Source: CAD feature listing. Evaluate the final solid. Frame: model axes, mm. Face numbers are marked on the shaded views. A direction names the side the tool comes from. Give positions to 0.01 mm unless a question says otherwise; leave off trailing zeros. Loops run counter-clockwise (first coordinate to the right, second up) from the corner with the lowest first, then second, coordinate; pieces in that order, holes last. Notation, with made-up numbers: M 16.5,-29.5 L 39.5,-29.5 A19 cw 39.5,-17.5 Z; hole C 28,77 d6. An arc over 180 degrees is marked long. Write item = value, one per line.
Solid Edge part; units mm, degrees
sketch "Sketch1" plane through (0, 0, 0) normal (0, 0, 1) x (1, 0, 0)
  circle A0 centre (0, 0) radius 3
extrude "Protrusion1" add sketch "Sketch1" along normal blind 37
sketch "Sketch2" plane through (0, 0, 37) normal (0, 0, 1) x (1, 0, 0)
  line L0 (-2.8847, 4.9965) -> (-5.7695, 0)
  line L1 (-5.7695, 0) -> (-2.8847, -4.9965)
  line L2 (-2.8847, -4.9965) -> (2.8847, -4.9965)
  line L3 (2.8847, -4.9965) -> (5.7695, 0)
  line L4 (5.7695, 0) -> (2.8847, 4.9965)
  line L5 (2.8847, 4.9965) -> (-2.8847, 4.9965)
extrude "ExtrudedProtrusion_2" add sketch "Sketch2" along normal blind 4
cosmetic_thread "Thread_1" thread depth 10
properties material "Steel"
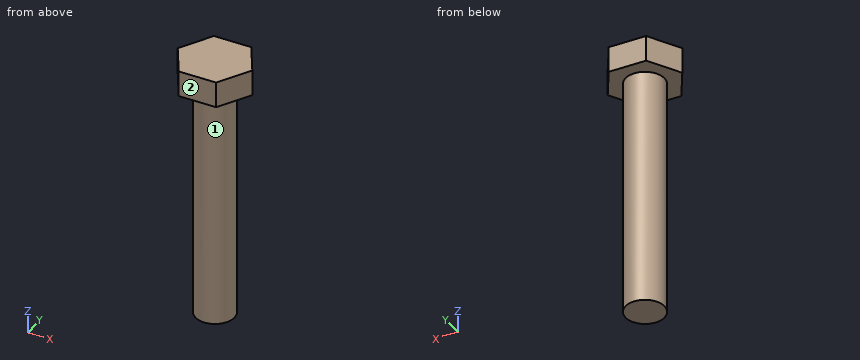
1. Cut plane D-D, the plane x = 5.25. Return the cut outline in (y, z), then the cut area to 3 significant figures.
Derived:
outline = M -0.9,37 L 0.9,37 L 0.9,41 L -0.9,41 Z
area = 7.20 mm²
2. Material intervals for probe 1 along Y at (x, z) = (0, 9); probe 2 along Z at (x, y) = (0.5, -3.25); probe 3 along X at (y, z) = (-2.75, 7.5), sorted ascending. Write a range as from..to.
Derived:
probe_1 = -3..3
probe_2 = 37..41
probe_3 = -1.2..1.2
3. First-contact query: pin 1 Ø4 at (x, z) = (-3.5, 14) entering from +Y; pin 2 Ø5 at (x, z) = (-3.5, 7) entering from -Y; pin 3 Ø1 at (y, z) = (0, 5.5) entering from -X. Flat tips, straight axial feed; report the tip coordinate or a pass-through.
Derived:
pin_1 = 2.6
pin_2 = -2.83
pin_3 = -3
4. Reachability of the marked faces 1 and 2 from +Z, -Z, +X, -X, +Y, -Y: full face, straight path, thin tool, end or side. Return the list, or none.
Derived:
face_1 = -Z
face_2 = +Z, -Z, +X, -X, -Y
5. Cut plane A-A, the plane y = 0.5. Return the cut outline in (x, z), then the cut area to 3 significant figures.
Derived:
outline = M -5.48,37 L -2.96,37 L -2.96,0 L 2.96,0 L 2.96,37 L 5.48,37 L 5.48,41 L -5.48,41 Z
area = 263 mm²
6. Cut plane C-C, the plane z = 20.5. Return the cut outline in (x, y), then the cut area to 3 significant figures.
Derived:
outline = C 0,0 d6
area = 28.3 mm²
7. Cut plane B-B, the plane x = 0. Return the cut outline in (y, z), then the cut area to 3 significant figures.
Derived:
outline = M -5,37 L -3,37 L -3,0 L 3,0 L 3,37 L 5,37 L 5,41 L -5,41 Z
area = 262 mm²
